```python
from build123d import *

# Parameters (mm, degrees)
F0_W     = 51.054
F0_H     = 6.604
F0_W_2   = 50.8
F0_H_2   = 4.7625
F1_DEPTH = 4.7625


with BuildPart() as f1:
    # F0 (on Front) → F1 (new body)
    with BuildSketch(Plane.XZ):
        Polygon((-127, 76.2), (-182.5625, 76.2), (-182.5625, -25.273), (-177.673, -25.273), (-177.673, -76.2), (177.673, -76.2), (177.673, -25.273), (182.5625, -25.273), (182.5625, 76.2), (127, 76.2), (76.2, 76.2), (25.4, 76.2), (-25.4, 76.2), (-76.2, 76.2), align=None)
        with Locations((-101.6, 15.875)):
            Rectangle(F0_W, F0_H, mode=Mode.SUBTRACT)
        with Locations((0, 15.875)):
            Rectangle(F0_W, F0_H, mode=Mode.SUBTRACT)
        with Locations((101.6, 15.875)):
            Rectangle(F0_W, F0_H, mode=Mode.SUBTRACT)
        with Locations((-101.6, 78.58125)):
            Rectangle(F0_W_2, F0_H_2)
        with Locations((0, 78.58125)):
            Rectangle(F0_W_2, F0_H_2)
        with Locations((101.6, 78.58125)):
            Rectangle(F0_W_2, F0_H_2)
    extrude(amount=F1_DEPTH)


solid = f1.part
```
Geometry: final body of the model. Coordinates: model frame, mm. Coordinates: 2 decimals unless noted, no trailing zeros. Order: outer loops, then holes, each group sorted by start corner. A loop starts at its lowest first (then second) coordinate and runs counter-clockwise, first axis right, second up. Notation, with made-up numbers: M 1,69.5 L 50,69.5 A29 ccw 50,92.5 Z; hole C 50.25,57 d3. An arc over 180 degrees is marked long. Answer in a Markdown table with one row per item. Add a question column.
Q1. Contact query for flat-ended pins moving along their axis: P1, Ø1.4, axis at x = 180.5, y = -1.5, coming from the -Z side; P2, Ø1.4, axis at x = -141, y = -1.5, coming from the +Z side; P3, Ø2.5, axis at y = -3, z = 79.5, coming from the +X side. Output: stop coordinate, or through.
Q2. Section query D-D on x = 37.5. Return the cut outline in (y, z), and give its area (3 significant figures).
Q3. Section query B-B on y = -2.2. Count the separate pieces of the cut face and the enclosed holes in it, and give its area (3 significant figures).
Q4. Line query: L1, parallel to X at y = -3.7, z = 19; L2, parallel to Z at x = 96, y = -3.15; L3, parallel to Z at x = -166.5, y = -2.6. Output: solid intervals per line, ascending.
Q5. Section query C-C on z = -62. Return the cut outline in (x, y), and give its area (3 significant figures).
Q6. Section query A-A on x = 101. Return the cut outline in (y, z), and give its area (3 significant figures).
Completed:
| question | item | result |
|---|---|---|
| 1 | P1 | stops at z = -25.27 |
| 1 | P2 | stops at z = 76.2 |
| 1 | P3 | stops at x = 127 |
| 2 | outline | M -4.76,-76.2 L 0,-76.2 L 0,76.2 L -4.76,76.2 Z |
| 2 | area | 726 mm2 |
| 3 | separate pieces | 1 |
| 3 | enclosed holes | 3 |
| 3 | area | 54,900 mm2 |
| 4 | L1 | x = -182.56 to -127.13, -76.07 to -25.53, 25.53 to 76.07, 127.13 to 182.56 |
| 4 | L2 | z = -76.2 to 12.57, 19.18 to 80.96 |
| 4 | L3 | z = -76.2 to 76.2 |
| 5 | outline | M -177.67,-4.76 L 177.67,-4.76 L 177.67,0 L -177.67,0 Z |
| 5 | area | 1,690 mm2 |
| 6 | outline | M -4.76,-76.2 L 0,-76.2 L 0,12.57 L -4.76,12.57 Z; M -4.76,19.18 L 0,19.18 L 0,80.96 L -4.76,80.96 Z |
| 6 | area | 717 mm2 |
